```python
from build123d import *

# Parameters (mm, degrees)
F1_DEPTH = 25.4
F3_D     = 12.7
F5_D     = 23.41626


with BuildPart() as f1:
    # F0 (on Front) → F1 (new body, symmetric)
    with BuildSketch(Plane.XZ):
        Polygon((-19.05, 31.75), (-31.75, 31.75), (-31.75, -31.75), (31.75, -31.75), (31.75, 31.75), (19.05, 31.75), (19.05, -6.35), (-19.05, -6.35), align=None)
    extrude(amount=F1_DEPTH, both=True)

    # F3 (through all)
    with Locations(Plane(origin=(-31.75, 0, 0), x_dir=(0, -1, 0), z_dir=(-1, 0, 0))):
        with Locations((0, 19.05)):
            Hole(F3_D / 2)

    # F5 (through all)
    with Locations(Plane.XY.offset(-6.35)):
        with Locations((0, 0)):
            Hole(F5_D / 2)


solid = f1.part
```
For this review, take the finished solid that the model builds, in its own axes (mm). A direction names the side the tool comes from. Round coordinates to 2 decimals unless told otherwise and drop trailing zeros. Write each loop counter-clockwise with the first axis right and the second up, starting at its lowest first coordinate (ties: lowest second). Pieces come first, ordered by that corner, then holes. Notation, with made-up numbers: (53, -24.5) -> (73, -24.5) arc R18 ccw to (73, -19.5) -> close; hole circle Ø2 at (12, 70). An arc over 180 degrees is marked (long way). One line per question, with ' | ' between items. Start each with the question number.
(1) For line 1 along X through (y, z) = (21.5, 6); line 2 along Y through (x, z) = (0, -21); line 3 along Z through (x, y) = (24, 0), list the stretches that pass through material, from the lowest coordinate up. Write a range as from..to.
(2) Insertion check: P1, Ø10, axis at y = 0, z = 19.05, coming from the +X side; P2, Ø19, axis at x = -1, y = 3.5, coming from the +Z side. Each pin has a flat end and moves straight along its axis. Give the tip position at first contact, or say it passes through.
(3) Tool access review of faces 1 (the face through (25.489, 3.414, 24.404)), 2 (the face through (-19.05, 0, 12)): name each direction out of +Z, -Z, +X, -X, +Y, -Y from which nothing blocks a thin tool from reaching the whole face with its end or side.
(4) Add section A-A, the plane x = 0. Write out the cut boundary in (y, z).
(5) Add section C-C, the plane y = 0. Write out the cut boundary in (x, z).
(6) Add section B-B, the plane z = 19.05. Write out the cut boundary in (x, y).
(7) Add section D-D, the plane z = 5.5. Write out the cut boundary in (x, y).
(8) Mouldability with a two-part tool opening along Y and no side actions: class faces 3 (the face through (-25, 0, 31.75)), 4 (the face through (0, 25.4, -7)), 5 (the face through (11.697, 0.515, -19.228)) as released by +Y, released by -Y, zero draft, split by the parting line, or undercut.
Answer list:
1) line 1: -31.75..-19.05, 19.05..31.75 | line 2: -25.4..-11.71, 11.71..25.4 | line 3: -31.75..12.7, 25.4..31.75
2) P1: through | P2: z = -6.35
3) face 1: +X, -X | face 2: +Z, +Y, -Y
4) outline: (-25.4, -31.75) -> (-11.71, -31.75) -> (-11.71, -6.35) -> (-25.4, -6.35) -> close; (11.71, -31.75) -> (25.4, -31.75) -> (25.4, -6.35) -> (11.71, -6.35) -> close
5) outline: (-31.75, -31.75) -> (-11.71, -31.75) -> (-11.71, -6.35) -> (-19.05, -6.35) -> (-19.05, 12.7) -> (-31.75, 12.7) -> close; (-31.75, 25.4) -> (-19.05, 25.4) -> (-19.05, 31.75) -> (-31.75, 31.75) -> close; (11.71, -31.75) -> (31.75, -31.75) -> (31.75, 12.7) -> (19.05, 12.7) -> (19.05, -6.35) -> (11.71, -6.35) -> close; (19.05, 25.4) -> (31.75, 25.4) -> (31.75, 31.75) -> (19.05, 31.75) -> close
6) outline: (-31.75, -25.4) -> (-19.05, -25.4) -> (-19.05, -6.35) -> (-31.75, -6.35) -> close; (-31.75, 6.35) -> (-19.05, 6.35) -> (-19.05, 25.4) -> (-31.75, 25.4) -> close; (19.05, -25.4) -> (31.75, -25.4) -> (31.75, -6.35) -> (19.05, -6.35) -> close; (19.05, 6.35) -> (31.75, 6.35) -> (31.75, 25.4) -> (19.05, 25.4) -> close
7) outline: (-31.75, -25.4) -> (-19.05, -25.4) -> (-19.05, 25.4) -> (-31.75, 25.4) -> close; (19.05, -25.4) -> (31.75, -25.4) -> (31.75, 25.4) -> (19.05, 25.4) -> close
8) face 3: zero draft | face 4: released by +Y | face 5: undercut
